```python
from build123d import *

# Parameters (mm, degrees)
SKETCH_1_W               = 98.8
SKETCH_1_H               = 96.2
EXTRUDE_2_DEPTH          = 15
CUT_EXTRUDE_1_DEPTH      = 43
CUT_EXTRUDE_1_DEPTH_BACK = 57
SKETCH_4_W               = 84.8
SKETCH_4_H               = 82.2
SKETCH_10_W              = 15
SKETCH_10_H              = 32.1
EXTRUDE_4_DEPTH          = 16
SKETCH_11_W              = 12.2
SKETCH_11_H              = 28.2
CUT_EXTRUDE_2_DEPTH      = 9
SKETCH_12_R              = 5.011519167
EXTRUDE_5_DEPTH          = 26.7
SKETCH_13_R              = 1.5
EXTRUDE_6_DEPTH          = 11.7
SKETCH_14_W              = 15
SKETCH_14_H              = 3.984812986
EXTRUDE_7_DEPTH          = 6.7
FILLET_1_R               = 10
SKETCH_15_W              = 1.4
SKETCH_15_H              = 28.115187014
EXTRUDE_8_DEPTH          = 6.7
SKETCH_17_W              = 1.4
SKETCH_17_H              = 28.115187014
EXTRUDE_9_DEPTH          = 6.7
CUT_EXTRUDE_3_DEPTH      = 128
CUT_EXTRUDE_3_DEPTH_BACK = 32.7
SKETCH_18_R              = 1.5
CUT_EXTRUDE_4_DEPTH      = 107
CUT_EXTRUDE_4_DEPTH_BACK = 39.7
SKETCH_19_R              = 1.5


with BuildPart() as part:
    # Эскиз1 → Бобышка-Вытянуть2 (new body)
    with BuildSketch(Plane.XY):
        with Locations((49.4, -48.1)):
            Rectangle(SKETCH_1_W, SKETCH_1_H)
    extrude(amount=EXTRUDE_2_DEPTH)

    # Эскиз4 → Вырез-Вытянуть1 (cut, two sides: drawn at the far end of the back side and taken through both)
    with BuildSketch(Plane.XY.offset(15).offset(-CUT_EXTRUDE_1_DEPTH_BACK)):
        with Locations((49.4, -48.1)):
            Rectangle(SKETCH_4_W, SKETCH_4_H)
    extrude(amount=CUT_EXTRUDE_1_DEPTH + CUT_EXTRUDE_1_DEPTH_BACK, mode=Mode.SUBTRACT)

    # Эскиз10 → Бобышка-Вытянуть4 (add)
    with BuildSketch(Plane(origin=(98.8, 0, 0), x_dir=(0, 0, -1), z_dir=(1, 0, 0))):
        with Locations((-7.5, -73.15)):
            Rectangle(SKETCH_10_W, SKETCH_10_H)
    extrude(amount=-EXTRUDE_4_DEPTH)

    # Эскиз11 → Вырез-Вытянуть2 (cut)
    with BuildSketch(Plane.ZY.offset(-82.8)):
        with Locations((7.5, -71.1)):
            Rectangle(SKETCH_11_W, SKETCH_11_H)
    extrude(amount=-CUT_EXTRUDE_2_DEPTH, mode=Mode.SUBTRACT)

    # Эскиз12 → Бобышка-Вытянуть5 (add)
    with BuildSketch(Plane.ZY.offset(-91.8)):
        with Locations((7.5, -39.6)):
            Circle(SKETCH_12_R)
    extrude(amount=EXTRUDE_5_DEPTH)

    # Эскиз13 → Бобышка-Вытянуть6 (add)
    with BuildSketch(Plane.ZY.offset(-65.1)):
        with Locations((7.5, -39.6)):
            Circle(SKETCH_13_R)
    extrude(amount=EXTRUDE_6_DEPTH)

    # Эскиз14 → Бобышка-Вытянуть7 (add)
    with BuildSketch(Plane.ZY.offset(-82.8)):
        with Locations((7.5, -87.207593507)):
            Rectangle(SKETCH_14_W, SKETCH_14_H)
    extrude(amount=EXTRUDE_7_DEPTH)

    # Скругление1
    # the kernel refuses this fillet: 10 mm, written as the material it takes off along each edge
    with BuildSketch(Plane(origin=(82.8, -85.2, 13.6), x_dir=(0, -1, 0), z_dir=(0, 0, -1))) as fillet_1_piece_1:
        with BuildLine():
            CenterArc((10, -0.550917082), FILLET_1_R, 176.841878722, 3.158121278)
            Line((0, -0.550917082), (0, 0))
            Line((0, 0), (0.015187014, 0))
        make_face()
    extrude(amount=12.2, mode=Mode.SUBTRACT)

    # Эскиз15 → Бобышка-Вытянуть8 (add)
    with BuildSketch(Plane.ZY.offset(-82.8)):
        with Locations((0.7, -71.157593507)):
            Rectangle(SKETCH_15_W, SKETCH_15_H)
    extrude(amount=EXTRUDE_8_DEPTH)

    # Эскиз17 → Бобышка-Вытянуть9 (add)
    with BuildSketch(Plane.ZY.offset(-82.8)):
        with Locations((14.3, -71.157593507)):
            Rectangle(SKETCH_17_W, SKETCH_17_H)
    extrude(amount=EXTRUDE_9_DEPTH)

    # Эскиз18 → Вырез-Вытянуть3 (cut, two sides: drawn at the far end of the back side and taken through both)
    with BuildSketch(Plane(origin=(7, 0, 0), x_dir=(0, 0, -1), z_dir=(1, 0, 0)).offset(-CUT_EXTRUDE_3_DEPTH_BACK)):
        with Locations(Location((-7.365603058, -49.501812711, 0), (0, 0, 180))):
            Circle(SKETCH_18_R)
    extrude(amount=CUT_EXTRUDE_3_DEPTH + CUT_EXTRUDE_3_DEPTH_BACK, mode=Mode.SUBTRACT)

    # Эскиз19 → Вырез-Вытянуть4 (cut, two sides: drawn at the far end of the back side and taken through both)
    with BuildSketch(Plane(origin=(0, -89.2, 0), x_dir=(1, 0, 0), z_dir=(0, 1, 0)).offset(-CUT_EXTRUDE_4_DEPTH_BACK)):
        with Locations((26.080914384, -7.5)):
            Circle(SKETCH_19_R)
    extrude(amount=CUT_EXTRUDE_4_DEPTH + CUT_EXTRUDE_4_DEPTH_BACK, mode=Mode.SUBTRACT)


solid = part.part
```
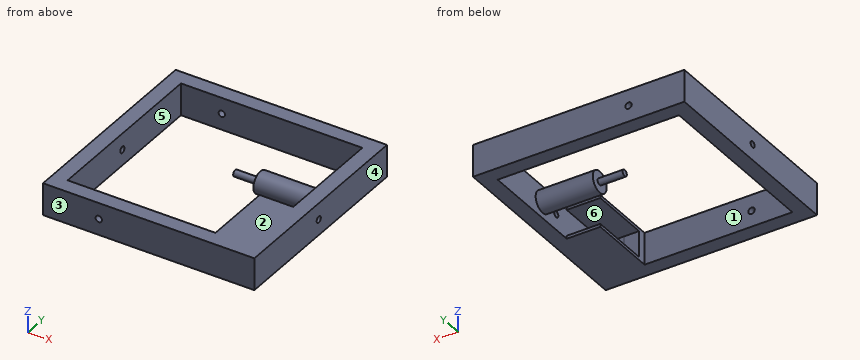
The listing builds one solid part. Answer for the finished solid, in the listing's coordinates (mm). Face numbers are marked on the shaded views. A direction names the side the tool comes from. Round coordinates to 2 decimals unless told otherwise and drop trailing zeros. Loops run counter-clockwise (first coordinate to the right, second up) from the corner with the lowest first, then second, coordinate; pieces in that order, holes last. Notation, with made-up numbers: (89.5, 10.5) - (115.5, 10.5) arc R27 ccw to (115.5, 28.5) - close; hole circle Ø8 at (20.5, 35). An arc over 180 degrees is marked (long way). Return JSON: item names as keys, results as strings. Group by question number.
1. The part is cut by section A-A on x = 84.5. Determine the outline of the cut face in (y, z), then the cut area to 3 significant figures.
2. The part is cut by section D-D on z = 3.75. Determine the outline of the cut face in (x, y), then the cut area to 3 significant figures.
3. The mould has two halves that part along Y. Classify the marked faces 1, 2 and 3: pulls with the +Y half, pulls with the -Y half, needs draft (parallel to the pull), parting line crosses it, or undercut.
4. Consider probe 1 along Y at (x, z) = (80, 7.5); probe 2 along X at (y, z) = (-73, 3.75); probe 3 along Y at (x, z) = (41, 3). Determine where each line is inside the solid, lowest interval first.
5. Which of the six approach directions +Z, -Z, +X, -X, +Y, -Y give full straight-line access (tool end or side, diameter ignored) to the marked faces 4, 5 and 6?
6. Each of these flat-tipped pins is pushed along its axis until it touches: P1, Ø12, axis at x = 66, y = -70.5, coming from the -Z side; P2, Ø10, axis at x = 51, y = -44, coming from the -Z side. Where does it stop, or does it pass through?
7. The part is cut by section C-C on y = -13.5. Determine the outline of the cut face in (x, z), then the cut area to 3 significant figures.
8. The part is cut by section B-B on y = -63. Determine the outline of the cut face in (x, z).
Resolved:
{
 "1": {"outline": "(-96.2, 0) - (-57.1, 0) - (-57.1, 1.4) - (-85.2, 1.4) - (-85.2, 13.6) - (-57.1, 13.6) - (-57.1, 15) - (-96.2, 15) - close; circle Ø10.02 at (-39.6, 7.5); (-7, 0) - (0, 0) - (0, 15) - (-7, 15) - close", "area": "428 mm²"},
 "2": {"outline": "(0, -96.2) - (98.8, -96.2) - (98.8, 0) - (0, 0) - close; hole (7, -89.2) - (76.1, -89.2) - (76.1, -85.22) - (82.8, -85.22) arc R10 cw to (83.35, -85.2) - (91.8, -85.2) - (91.8, -42.92) - (65.1, -42.92) - (65.1, -36.28) - (91.8, -36.28) - (91.8, -7) - (7, -7) - close", "area": "2,770 mm²"},
 "3": {"face 1": "undercut", "face 2": "needs draft", "face 3": "pulls with the -Y half"},
 "4": {"probe 1": "y = -96.2 to -85.22, -44.61 to -34.59, -7 to 0", "probe 2": "x = 0 to 7, 91.8 to 98.8", "probe 3": "y = -96.2 to -89.2, -7 to 0"},
 "5": {"face 4": "+Z, -Z, +X, +Y, -Y", "face 5": "+Z, -Z", "face 6": "none"},
 "6": {"P1": "passes through", "P2": "stops at z = 6"},
 "7": {"outline": "(0, 0) - (7, 0) - (7, 15) - (0, 15) - close; (91.8, 0) - (98.8, 0) - (98.8, 15) - (91.8, 15) - close", "area": "210 mm²"},
 "8": {"outline": "(0, 0) - (7, 0) - (7, 15) - (0, 15) - close; (76.1, 0) - (98.8, 0) - (98.8, 15) - (76.1, 15) - (76.1, 13.6) - (91.8, 13.6) - (91.8, 1.4) - (76.1, 1.4) - close"}
}
